from build123d import *

# Parameters (mm, degrees)
F0_R     = 1.5875
F1_DEPTH = 3.175


with BuildPart() as f1:
    # F0 (on Top) → F1 (new body)
    with BuildSketch(Plane.XY):
        with BuildLine():
            ThreePointArc((48.298852367, 25.3648877175), (46.5534190331, 34.1258622353), (41.5836577474, 41.5489805011))
            ThreePointArc((41.5836577474, 41.5489805011), (25.5683959748, 48.2245206641), (9.478505781, 41.7309176838))
            ThreePointArc((9.478505781, 41.7309176838), (9.2940469865, 9.1807949339), (41.8436252726, 9.4443655555))
            ThreePointArc((41.8436252726, 9.4443655555), (46.6236666053, 16.7751702782), (48.298852367, 25.3648877175))
        make_face()
        with BuildLine():
            ThreePointArc((19.088852367, 11.0773877175), (16.3788203518, 9.9548557024), (17.501352367, 12.6648877175))
            ThreePointArc((17.501352367, 12.6648877175), (18.6238843821, 12.1999197327), (19.088852367, 11.0773877175))
        make_face(mode=Mode.SUBTRACT)
        with Locations((9.525, 31.75)):
            Circle(F0_R, mode=Mode.SUBTRACT)
        with BuildLine():
            Line((38.1080227106, 38.0648877175), (38.138852367, 38.0648877175))
            Line((38.138852367, 38.0648877175), (38.138852367, 12.6648877175))
            Line((38.138852367, 12.6648877175), (33.669537083, 12.6648877175))
            ThreePointArc((33.669537083, 12.6648877175), (34.5718551189, 12.110760332), (34.925, 11.1125))
            ThreePointArc((34.925, 11.1125), (32.339239668, 9.8781448811), (33.005462917, 12.6648877175))
            Line((33.005462917, 12.6648877175), (17.501352367, 12.6648877175))
            Line((17.501352367, 12.6648877175), (12.738852367, 12.6648877175))
            Line((12.738852367, 12.6648877175), (12.738852367, 38.0648877175))
            Line((12.738852367, 38.0648877175), (38.1080227106, 38.0648877175))
        make_face(mode=Mode.SUBTRACT)
        with Locations((41.275, 31.75)):
            Circle(F0_R, mode=Mode.SUBTRACT)
        with BuildLine():
            Line((57.9526965359, 57.9578523511), (41.5836577474, 41.5489805011))
            ThreePointArc((41.5836577474, 41.5489805011), (46.5534190331, 34.1258622353), (48.298852367, 25.3648877175))
            ThreePointArc((48.298852367, 25.3648877175), (46.6236666053, 16.7751702782), (41.8436252726, 9.4443655555))
            add(Edge.make_bspline(
                [(86.8310062503, 56.0153192292), (83.249706502, 51.2144143314), (63.5484661138, 26.0258843806), (51.3080659428, 17.112891847), (41.8436252726, 9.4443655555)],
                knots=[0.7406020956, 0.7406020956, 0.7406020956, 0.7406020956, 0.7871603002, 1, 1, 1, 1], degree=3))
            ThreePointArc((86.8310062503, 56.0153192292), (75.7950461349, 59.6100245839), (66.4012027896, 66.4269175316))
            Line((66.4012027896, 66.4269175316), (60.1950306165, 60.2056430155))
            ThreePointArc((60.1950306165, 60.2056430155), (60.540152928, 59.6901486915), (60.6613635762, 59.0817476833))
            ThreePointArc((60.6613635762, 59.0817476833), (59.6822645844, 57.6154583315), (57.9526965359, 57.9578523511))
        make_face()
        with BuildLine():
            ThreePointArc((9.478505781, 41.7309176838), (25.5683959748, 48.2245206641), (41.5836577474, 41.5489805011))
            Line((41.5836577474, 41.5489805011), (57.9526965359, 57.9578523511))
            ThreePointArc((57.9526965359, 57.9578523511), (57.949968244, 60.2029147236), (60.1950306165, 60.2056430155))
            Line((60.1950306165, 60.2056430155), (66.4012027896, 66.4269175316))
            ThreePointArc((66.4012027896, 66.4269175316), (59.7830008839, 75.3788925735), (56.1057766209, 85.88681698))
            add(Edge.make_bspline(
                [(9.478505781, 41.7309176838), (17.0929440337, 51.1603431722), (26.371548526, 62.5901940603), (51.3329129213, 82.2718852167), (56.1057766209, 85.88681698)],
                knots=[0, 0, 0, 0, 0.211634739, 0.2581952867, 0.2581952867, 0.2581952867, 0.2581952867], degree=3))
        make_face()
        with BuildLine():
            Line((89.1799820166, 89.261127534), (66.4012027896, 66.4269175316))
            ThreePointArc((66.4012027896, 66.4269175316), (75.7950461349, 59.6100245839), (86.8310062503, 56.0153192292))
            add(Edge.make_bspline(
                [(113.9930376147, 98.1438093202), (107.5652173309, 85.5841385514), (97.0153094729, 69.6678684875), (86.8310062503, 56.0153192292)],
                knots=[0.6082024344, 0.6082024344, 0.6082024344, 0.6082024344, 0.7406020956, 0.7406020956, 0.7406020956, 0.7406020956], degree=3))
            Line((113.9930376147, 98.1438093202), (105.9976837923, 106.1197541654))
            Line((105.9976837923, 106.1197541654), (96.2377675544, 96.3360877642))
            ThreePointArc((96.2377675544, 96.3360877642), (97.3240460353, 94.7135604092), (97.7055586597, 92.7986076491))
            ThreePointArc((97.7055586597, 92.7986076491), (94.6238275456, 88.1834363993), (89.1799820166, 89.261127534))
        make_face()
        with BuildLine():
            add(Edge.make_bspline(
                [(56.1057766209, 85.88681698), (69.7989441385, 96.2579210625), (85.7273267139, 107.1699447817), (98.2606169463, 113.8380390341)],
                knots=[0.2581952867, 0.2581952867, 0.2581952867, 0.2581952867, 0.3917757571, 0.3917757571, 0.3917757571, 0.3917757571], degree=3))
            ThreePointArc((56.1057766209, 85.88681698), (59.7830008839, 75.3788925735), (66.4012027896, 66.4269175316))
            Line((66.4012027896, 66.4269175316), (89.1799820166, 89.261127534))
            ThreePointArc((89.1799820166, 89.261127534), (89.1713946704, 96.327500418), (96.2377675544, 96.3360877642))
            Line((96.2377675544, 96.3360877642), (105.9976837923, 106.1197541654))
            Line((105.9976837923, 106.1197541654), (98.2606169463, 113.8380390341))
        make_face()
        with BuildLine():
            Line((38.138852367, 12.6648877175), (38.138852367, 38.0648877175))
            Line((38.138852367, 38.0648877175), (38.1080227106, 38.0648877175))
            Line((38.1080227106, 38.0648877175), (12.738852367, 38.0648877175))
            Line((12.738852367, 38.0648877175), (12.738852367, 12.6648877175))
            Line((12.738852367, 12.6648877175), (17.501352367, 12.6648877175))
            Line((17.501352367, 12.6648877175), (33.005462917, 12.6648877175))
            ThreePointArc((33.005462917, 12.6648877175), (33.3375, 12.7), (33.669537083, 12.6648877175))
            Line((33.669537083, 12.6648877175), (38.138852367, 12.6648877175))
        make_face()
        with BuildLine():
            ThreePointArc((33.6445749551, 25.3648877175), (17.8596626631, 22.2200877834), (31.2341189545, 31.1742567343))
            ThreePointArc((31.2341189545, 31.1742567343), (33.0180420708, 28.5096876517), (33.6445749551, 25.3648877175))
        make_face(mode=Mode.SUBTRACT)
        with BuildLine():
            Line((105.9976837923, 106.1197541654), (113.9930376147, 98.1438093202))
            add(Edge.make_bspline(
                [(119.0607801069, 119.1260976819), (121.7354589285, 116.3963605732), (119.2349256659, 108.3862220235), (113.9930376147, 98.1438093202)],
                knots=[0.5002304981, 0.5002304981, 0.5002304981, 0.5002304981, 0.6082024344, 0.6082024344, 0.6082024344, 0.6082024344], degree=3))
            ThreePointArc((119.0607801069, 119.1260976819), (119.038672719, 119.1482070061), (119.0165467814, 119.1702977666))
            Line((119.0165467814, 119.1702977666), (105.9976837923, 106.1197541654))
        make_face()
        with BuildLine():
            add(Edge.make_bspline(
                [(98.2606169463, 113.8380390341), (108.3812043908, 119.2225015111), (116.2880200857, 121.8397075452), (119.0165467814, 119.1702977666)],
                knots=[0.3917757571, 0.3917757571, 0.3917757571, 0.3917757571, 0.4996415136, 0.4996415136, 0.4996415136, 0.4996415136], degree=3))
            Line((98.2606169463, 113.8380390341), (105.9976837923, 106.1197541654))
            Line((105.9976837923, 106.1197541654), (119.0165467814, 119.1702977666))
        make_face()
        with BuildLine():
            Line((132.9733085625, 133.1610224797), (119.0165467814, 119.1702977666))
            add(Edge.make_bspline(
                [(119.0165467814, 119.1702977666), (119.0314454842, 119.1557218627), (119.0461897944, 119.1409883361), (119.0607801069, 119.1260976819)],
                knots=[0.4996415136, 0.4996415136, 0.4996415136, 0.4996415136, 0.5002304981, 0.5002304981, 0.5002304981, 0.5002304981], degree=3))
            ThreePointArc((119.0607801069, 119.1260976819), (121.0771249041, 116.9399007111), (122.9126341528, 114.5998132483))
            Line((122.9126341528, 114.5998132483), (132.9733085625, 133.1610224797))
        make_face()
        with BuildLine():
            Line((132.9733085625, 133.1610224797), (114.6029810942, 122.9350930852))
            ThreePointArc((114.6029810942, 122.9350930852), (116.8831644106, 121.1387446745), (119.0165467814, 119.1702977666))
            Line((119.0165467814, 119.1702977666), (132.9733085625, 133.1610224797))
        make_face()
        with BuildLine():
            ThreePointArc((96.2377675544, 96.3360877642), (89.1713946704, 96.327500418), (89.1799820166, 89.261127534))
            Line((89.1799820166, 89.261127534), (91.5877077452, 91.6747123169))
            ThreePointArc((91.5877077452, 91.6747123169), (91.5849794533, 93.9197746894), (93.8300418258, 93.9225029813))
            Line((93.8300418258, 93.9225029813), (96.2377675544, 96.3360877642))
        make_face()
        with BuildLine():
            Line((91.5877077452, 91.6747123169), (89.1799820166, 89.261127534))
            ThreePointArc((89.1799820166, 89.261127534), (94.6238275456, 88.1834363993), (97.7055586597, 92.7986076491))
            ThreePointArc((97.7055586597, 92.7986076491), (97.3240460353, 94.7135604092), (96.2377675544, 96.3360877642))
            Line((96.2377675544, 96.3360877642), (93.8300418258, 93.9225029813))
            ThreePointArc((93.8300418258, 93.9225029813), (94.1751641373, 93.4070086573), (94.2963747855, 92.7986076491))
            ThreePointArc((94.2963747855, 92.7986076491), (93.3172757937, 91.3323182973), (91.5877077452, 91.6747123169))
        make_face()
        with BuildLine():
            add(Edge.make_bspline(
                [(119.0607801069, 119.1260976819), (121.7354589285, 116.3963605732), (119.2349256659, 108.3862220235), (113.9930376147, 98.1438093202)],
                knots=[0.5002304981, 0.5002304981, 0.5002304981, 0.5002304981, 0.6082024344, 0.6082024344, 0.6082024344, 0.6082024344], degree=3))
            Line((113.9930376147, 98.1438093202), (122.9126341528, 114.5998132483))
            ThreePointArc((122.9126341528, 114.5998132483), (121.0771249041, 116.9399007111), (119.0607801069, 119.1260976819))
        make_face()
        with BuildLine():
            ThreePointArc((119.0165467814, 119.1702977666), (116.8831644106, 121.1387446745), (114.6029810942, 122.9350930852))
            Line((114.6029810942, 122.9350930852), (98.2606169463, 113.8380390341))
            add(Edge.make_bspline(
                [(98.2606169463, 113.8380390341), (108.3812043908, 119.2225015111), (116.2880200857, 121.8397075452), (119.0165467814, 119.1702977666)],
                knots=[0.3917757571, 0.3917757571, 0.3917757571, 0.3917757571, 0.4996415136, 0.4996415136, 0.4996415136, 0.4996415136], degree=3))
        make_face()
        with BuildLine():
            add(Edge.make_bspline(
                [(119.0165467814, 119.1702977666), (119.0314454842, 119.1557218627), (119.0461897944, 119.1409883361), (119.0607801069, 119.1260976819)],
                knots=[0.4996415136, 0.4996415136, 0.4996415136, 0.4996415136, 0.5002304981, 0.5002304981, 0.5002304981, 0.5002304981], degree=3))
            ThreePointArc((119.0165467814, 119.1702977666), (119.038672719, 119.1482070061), (119.0607801069, 119.1260976819))
        make_face()
    extrude(amount=F1_DEPTH)


solid = f1.part
Work out the finished part from the listing and answer in its coordinate system (mm). Give positions to 0.01 mm unless a question says otherwise; leave off trailing zeros. Order: outer loops, then holes, each group sorted by start corner. A loop starts at its lowest first (then second) coordinate and runs counter-clockwise, first axis right, second up. Notation, with made-up numbers: (27, 9) - (43, 9) arc R24 ccw to (43, 33) - close; hole circle Ø6 at (-2, 73). An arc over 180 degrees is marked (long way). Answer as CSV lines item,"result". Start each with the question number.
Q1. The part is cut by section A-A (z = 1.05). Give the number of separate pieces and of enclosed holes in the cut face, then the cut area to 3 significant figures.
Q2. Find the intervals of material crossed by L1, parallel to Y at x = 20, z = 3; L2, parallel to Y at x = 27.5, z = 2.5; L3, parallel to X at y = 81, z = 1.8, in increasing order. Write a range as [from, to].
Q3. The mould has two halves that part along Y. Classify faces 1 (the face through (115.86, 123.635, 1.565)), 2 (the face through (42.128, 33.089, 1.565)), 3 (the face through (67, 54, 3.175)), 4 (the face through (8.35, 32.82, 1.57)): +Y half, -Y half, draft (parallel to the pull), parting line (faces both ways), or undercut.
Q4. The part is cut by section B-B (x = 124.5). Write down the section's boundary in (y, z) (3 decimals).
Q5. Given pin 1 Ø1 at (x, z) = (64.5, 3) entering from -Y; pin 2 Ø1.5 at (x, z) = (111, 0.5) entering from -Y, each flat-ended and moving along its own axis, determine where each tip first touches the part or whether it passes through.
Check result:
1,separate pieces,"1"
1,enclosed holes,"7"
1,area,"5,720 mm²"
2,L1,"y = [3.16, 19.22], [31.51, 54.16]"
2,L2,"y = [2.6, 17.42], [33.31, 61.86]"
2,L3,"x = [49.77, 104.07]"
3,face 1,"+Y half"
3,face 2,"undercut"
3,face 3,"draft"
3,face 4,"undercut"
4,outline,"(117.528, 0) - (128.444, 0) - (128.444, 3.175) - (117.528, 3.175) - close"
5,pin 1,"stops at y = 28.81"
5,pin 2,"stops at y = 91.25"
